Part print with two shaded views. Sizes in mm from the minimum x, y, z corner. A direction names the side the tool comes from. Round coordinates to 2 decimals unless told otherwise and drop trailing zeros. Order: outer loops, then holes, each group sorted by start corner. A loop starts at its lowest first (then second) coordinate and runs counter-clockwise, first axis right, second up. Notation, with made-up numbers: (85, 70.5) -> (102, 70.5) arc R15 cw to (102, 99.5) -> close; hole circle Ø5 at (59.5, 72.5). An arc over 180 degrees is marked (long way). Put each result on its own line as item: value. Start each with the question number.
Q1. Probe L1, parallel to X at y = 10.25, z = 43; L2, parallel to Y at x = 71.5, z = 13.5. List the from-to ranges inside material, lowest first.
Q2. Pull direction Z, two halves, no side cores. Call the marked faces 1, 2, 3 and 4: released by +Z, released by -Z, zero draft, split by the parting line, or undercut.
Q3. Cut at C-C, the plane y = 14.25. List the corners of the cut face in (x, z), and give its area (3 significant figures).
Q4. Cut at B-B, the plane z = 24.5. List the corners of the cut face in (x, y).
Q5. 3-axis set-ups, long thin cutter, end or side, ignore diameter. For the marked faces 5 and 6: which of +Z, -Z, +X, -X, +Y, -Y reach the whole face in a straight line?
Q6. Cut at A-A, the plane x = 47. List the corners of the cut face in (y, z), and give its area (3 significant figures).
Q7. Flat gauge pins, fed straight in: P1, Ø6, axis at x = 79.5, y = 16, coming from the -Z side; P2, Ø10, axis at x = 17, z = 44, coming from the +Y side; P3, Ø1, axis at x = 41, z = 89, coming from the -Y side. Where does each tip first touch, or does it go through?
Q8. Cut at D-D, the plane x = 71. List the corners of the cut face in (y, z).
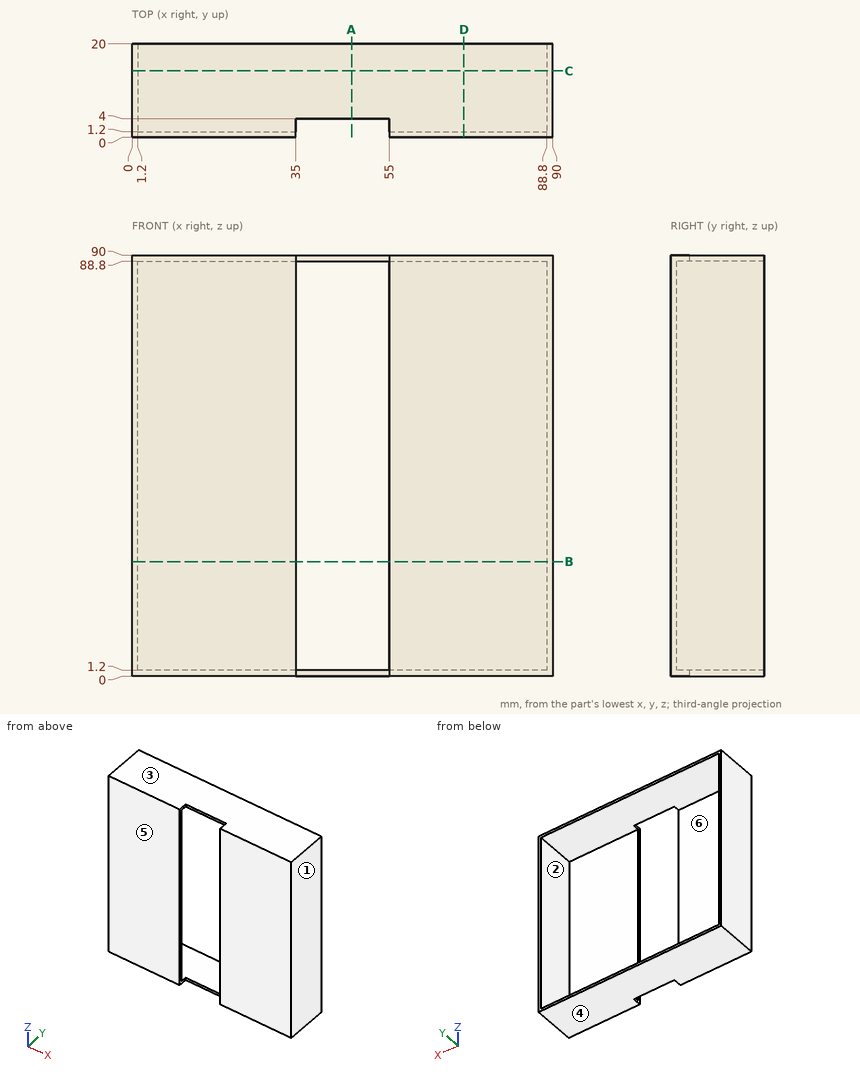
Ans:
1. L1: x = 0 to 1.2, 88.8 to 90
1. L2: y = 0 to 1.2
2. face 1: zero draft
2. face 2: undercut
2. face 3: released by +Z
2. face 4: released by -Z
3. outline: (0, 0) -> (90, 0) -> (90, 90) -> (0, 90) -> close; hole (1.2, 1.2) -> (88.8, 1.2) -> (88.8, 88.8) -> (1.2, 88.8) -> close
3. area: 426 mm^2
4. outline: (0, 0) -> (35, 0) -> (35, 1.2) -> (1.2, 1.2) -> (1.2, 20) -> (0, 20) -> close; (55, 0) -> (90, 0) -> (90, 20) -> (88.8, 20) -> (88.8, 1.2) -> (55, 1.2) -> close
5. face 5: +Z, -Z, +X, -X, -Y
5. face 6: +Y
6. outline: (4, 0) -> (20, 0) -> (20, 1.2) -> (4, 1.2) -> close; (4, 88.8) -> (20, 88.8) -> (20, 90) -> (4, 90) -> close
6. area: 38.4 mm^2
7. P1: stops at z = 0
7. P2: stops at y = 1.2
7. P3: stops at y = 4
8. outline: (0, 0) -> (20, 0) -> (20, 1.2) -> (1.2, 1.2) -> (1.2, 88.8) -> (20, 88.8) -> (20, 90) -> (0, 90) -> close
